Input: part model. Units: mm. Frame: model coordinates. A direction names the side the tool comes from. Coordinates: 2 decimals unless noted, no trailing zeros. Order: outer loops, then holes, each group sorted by start corner. A loop starts at its lowest first (then second) coordinate and runs counter-clockwise, first axis right, second up. Notation, with made-up numbers: (48, 25.5) -> (100, 25.5) arc R9 cw to (100, 35.5) -> close; hole circle Ø8 at (41, -13). An arc over 180 degrees is marked (long way). Answer as CSV lines item,"result".
from build123d import *

# Parameters (mm, degrees)
F0_W     = 15.8
F0_H     = 15.8
F1_DEPTH = 9.8
F2_R     = 2.45
F3_DEPTH = 1.83
F4_R     = 0.1


with BuildPart() as f1:
    # F0 (on Front) → F1 (new body)
    with BuildSketch(Plane.XZ):
        with Locations((10.663698, 7.9)):
            Rectangle(F0_W, F0_H)
    extrude(amount=F1_DEPTH)

    # F2 (on Front) → F3 (join)
    with BuildSketch(Plane.XZ):
        with Locations((6.688698, 11.875)):
            Circle(F2_R)
        with Locations((14.638698, 11.875)):
            Circle(F2_R)
        with Locations((6.688698, 3.925)):
            Circle(F2_R)
        with Locations((14.638698, 3.925)):
            Circle(F2_R)
    extrude(amount=-F3_DEPTH)

    # F4
    f4_edges = [f1.edges().sort_by_distance(p)[0] for p in [
        (12.188698, 1.83, 11.875),
        (4.238698, 1.83, 11.875),
        (4.238698, 1.83, 3.925),
        (12.188698, 1.83, 3.925),
    ]]
    fillet(f4_edges, radius=F4_R)


solid = f1.part
1. Cut plane B-B (y = 0.25). Return the cut outline in (x, z) (3 decimals).
Findings:
outline,"circle Ø4.9 at (6.689, 3.925); circle Ø4.9 at (6.689, 11.875); circle Ø4.9 at (14.639, 3.925); circle Ø4.9 at (14.639, 11.875)"
2. Cut plane C-C (z = 7). Return the cut outline in (x, y), plus the area to 3 significant figures.
Findings:
outline,"(2.76, -9.8) -> (18.56, -9.8) -> (18.56, 0) -> (2.76, 0) -> close"
area,"155 mm2"
3. Reachability of faces 4 (the face through (12.19, 0.85, 4.03)), 5 (the face through (11, -5, 15.8)) from +Z, -Z, +X, -X, +Y, -Y: full face, straight path, thin tool, end or side. Return the list, or none.
Findings:
face 4,"+Y"
face 5,"+Z, +X, -X, +Y, -Y"
4. Mould query, pull axis Z, two halves, no side actions, for faces 1 (the face through (8.01, 0.85, 5.99)), 2 (the face through (11, -5, 0)), 3 (the face through (15, 1.83, 4)). Classes: released by +Z, released by -Z, zero draft, split by the parting line, or undercut.
Findings:
face 1,"undercut"
face 2,"released by -Z"
face 3,"zero draft"
5. Ray query, line 1 along X through (y, z) = (0.5, 11.75); line 2 along Y through (x, z) = (12.5, 9.5); line 3 along X through (y, z) = (0.75, 4.75). Return the intervals inside material, ascending.
Findings:
line 1,"x = 4.24 to 9.14, 12.19 to 17.09"
line 2,"y = -9.8 to 0"
line 3,"x = 4.38 to 9, 12.33 to 16.95"
6. Cut plane A-A (x = 10.25). Return the cut outline in (y, z), plus the area to 3 significant figures.
Findings:
outline,"(-9.8, 0) -> (0, 0) -> (0, 15.8) -> (-9.8, 15.8) -> close"
area,"155 mm2"
